Geometry: final body of the model. Coordinates: model frame, mm. Give positions to 0.01 mm unless a question says otherwise; leave off trailing zeros. Loops run counter-clockwise (first coordinate to the right, second up) from the corner with the lowest first, then second, coordinate; pieces in that order, holes last. Notation, with made-up numbers: (74, 75) - (96, 75) arc R14 cw to (96, 85) - close; hole circle Ø2 at (8, 51). An arc over 180 degrees is marked (long way). Answer in a Markdown table with one row per item.
from build123d import *

# Parameters (mm, degrees)
SCHIZZO1_R                   = 17
SCHIZZO1_R_2                 = 2
SCHIZZO1_R_3                 = 4.5
SCHIZZO1_R_4                 = 1.5
ESTRUSIONE_ESTRUSIONE1_DEPTH = 10


with BuildPart() as part:
    # Schizzo1 → Estrusione-Estrusione1 (new body)
    with BuildSketch(Plane.XY):
        Polygon((2, 0), (448, 0), (450, 2), (450, 98), (448, 100), (2, 100), (0, 98), (0, 2), align=None)
        with Locations((225, 50)):
            Circle(SCHIZZO1_R, mode=Mode.SUBTRACT)
        with Locations(Location((239.849242405, 64.849242405, 0), (0, 0, 180))):
            Circle(SCHIZZO1_R_2, mode=Mode.SUBTRACT)
        with Locations(Location((104, 40.5, 0), (0, 0, 180))):
            Circle(SCHIZZO1_R_3, mode=Mode.SUBTRACT)
        with Locations((239.849242405, 35.150757595)):
            Circle(SCHIZZO1_R_2, mode=Mode.SUBTRACT)
        with Locations(Location((210.150757595, 35.150757595, 0), (0, 0, 180))):
            Circle(SCHIZZO1_R_2, mode=Mode.SUBTRACT)
        with Locations(Location((104, 80.5, 0), (0, 0, 180))):
            Circle(SCHIZZO1_R_3, mode=Mode.SUBTRACT)
        with Locations(Location((386, 40.5, 0), (0, 0, 180))):
            Circle(SCHIZZO1_R_3, mode=Mode.SUBTRACT)
        with Locations((64, 40.5)):
            Circle(SCHIZZO1_R_3, mode=Mode.SUBTRACT)
        with Locations((64, 80.5)):
            Circle(SCHIZZO1_R_3, mode=Mode.SUBTRACT)
        with Locations((346, 40.5)):
            Circle(SCHIZZO1_R_3, mode=Mode.SUBTRACT)
        with Locations((15, 30)):
            Circle(SCHIZZO1_R_4, mode=Mode.SUBTRACT)
        with Locations(Location((435, 30, 0), (0, 0, 180))):
            Circle(SCHIZZO1_R_4, mode=Mode.SUBTRACT)
        with Locations((210.150757595, 64.849242405)):
            Circle(SCHIZZO1_R_2, mode=Mode.SUBTRACT)
        with Locations((346, 80.5)):
            Circle(SCHIZZO1_R_3, mode=Mode.SUBTRACT)
        with Locations(Location((386, 80.5, 0), (0, 0, 180))):
            Circle(SCHIZZO1_R_3, mode=Mode.SUBTRACT)
        with Locations((435, 70)):
            Circle(SCHIZZO1_R_4, mode=Mode.SUBTRACT)
        with Locations(Location((15, 70, 0), (0, 0, 180))):
            Circle(SCHIZZO1_R_4, mode=Mode.SUBTRACT)
    extrude(amount=-ESTRUSIONE_ESTRUSIONE1_DEPTH)


solid = part.part
Q1. Cut plane C-C (z = -8.5). Give the number of separate pieces and of enclosed holes in the cut face, and give its area (3 significant figures).
Check values:
| item | result |
|---|---|
| separate pieces | 1 |
| enclosed holes | 17 |
| area | 43,500 mm² |
Q2. Cut plane B-B (y = 50). Output: boundary loops of the cut face in (x, z).
Check values:
| item | result |
|---|---|
| outline | (0, -10) - (208, -10) - (208, 0) - (0, 0) - close; (242, -10) - (450, -10) - (450, 0) - (242, 0) - close |
Q3. Material intervals for line 1 along Y through (x, z) = (386, -6.25); line 2 along X through (y, z) = (83, -2.25); line 3 along X through (y, z) = (38, -7), sorted ascending.
Check values:
| item | result |
|---|---|
| line 1 | 0 to 36, 45 to 76, 85 to 100 |
| line 2 | 0 to 60.26, 67.74 to 100.26, 107.74 to 342.26, 349.74 to 382.26, 389.74 to 450 |
| line 3 | 0 to 60.26, 67.74 to 100.26, 107.74 to 212.96, 237.04 to 342.26, 349.74 to 382.26, 389.74 to 450 |
Q4. Draft query along X for faces 1 (the flat face through (222, 73, -10)), 2 (the cylindrical face through (348.419, 84.294, -4.93)), 3 (the flat face through (0, 51, -5)). Return one class per face: pulls with the +X half, pulls with the -X half, needs draft (parallel to the pull), parting line crosses it, or undercut.
Check values:
| item | result |
|---|---|
| face 1 | needs draft |
| face 2 | undercut |
| face 3 | pulls with the -X half |
Q5. Cut plane A-A (x = 104). Output: boundary loops of the cut face in (y, z), and give its area (3 significant figures).
Check values:
| item | result |
|---|---|
| outline | (0, -10) - (36, -10) - (36, 0) - (0, 0) - close; (45, -10) - (76, -10) - (76, 0) - (45, 0) - close; (85, -10) - (100, -10) - (100, 0) - (85, 0) - close |
| area | 820 mm² |
